CAD build for the part. Positions are in the model's coordinates, mm. Face numbers are marked on the shaded views. A direction names the side the tool comes from. Coordinates: 2 decimals unless noted, no trailing zeros. Loops run counter-clockwise (first coordinate to the right, second up) from the corner with the lowest first, then second, coordinate; pieces in that order, holes last. Notation, with made-up numbers: (67, 55) -> (103, 55) arc R18 cw to (103, 84) -> close; hole circle Ø2 at (7, 16). An arc over 180 degrees is marked (long way). Answer as a JSON object with one key per item and string values. Group by question number.
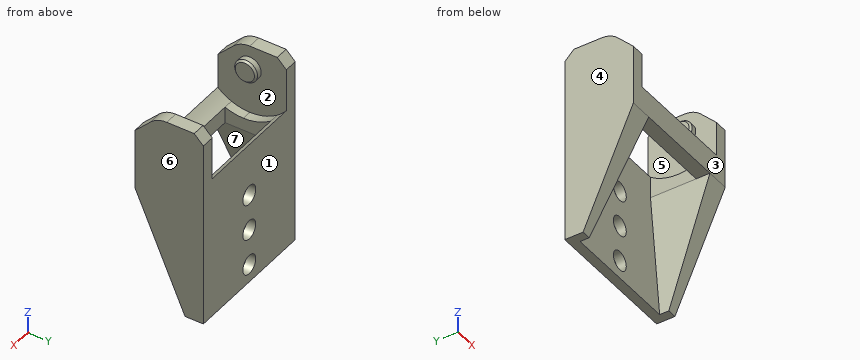
from build123d import *

# Parameters (mm, degrees)
SKETCH_1_W               = 30
SKETCH_1_H               = 15
EXTRUDE_1_DEPTH          = 18
CUT_EXTRUDE_1_REACH      = 28.843
SKETCH_2_W               = 20
SKETCH_2_H               = 10
CUT_EXTRUDE_2_REACH      = 29.668
SKETCH_3_W               = 20
SKETCH_3_H               = 12
CUT_EXTRUDE_5_DEPTH      = 22.1
CUT_EXTRUDE_5_DEPTH_BACK = 2.1
SKETCH_4_W               = 5
SKETCH_4_H               = 6
SKETCH_5_R               = 2.5
EXTRUDE_2_DEPTH          = 1.6
EXTRUDE_START            = 1.6
SKETCH_6_R               = 2.5
EXTRUDE_3_DEPTH          = 1.6
CHAMFER_1_SIZE           = 0.4
CUT_EXTRUDE_6_DEPTH      = 35.020684023
CUT_EXTRUDE_6_DEPTH_BACK = 35.020684023
CUT_EXTRUDE_7_DEPTH      = 35.020684023
CUT_EXTRUDE_7_DEPTH_BACK = 35.020684023
CHAMFER_2_SIZE           = 2
EXTRUDE_4_DEPTH          = 25
CHAMFER_3_SIZE           = 25
CHAMFER_3_SIZE2          = 11
SKETCH_10_R              = 2.1
CUT_EXTRUDE_8_DEPTH      = 15
CHAMFER_4_SIZE           = 3
CHAMFER_4_SIZE_2         = 25


with BuildPart() as part:
    # 草圖1 → 填料-伸長1 (new body)
    with BuildSketch(Plane.XY):
        with Locations((2.249045701, -2.44972067)):
            Rectangle(SKETCH_1_W, SKETCH_1_H)
    extrude(amount=EXTRUDE_1_DEPTH)

    # 草圖2 → 除料-伸長1 (cut, up to next)
    with BuildSketch(Plane.XY.offset(18), mode=Mode.PRIVATE) as cut_extrude_1_sk1:
        with Locations((2.249045701, -1.94972067)):
            Rectangle(SKETCH_2_W, SKETCH_2_H)
    cut_extrude_1_tool1 = extrude(cut_extrude_1_sk1.sketch, amount=-CUT_EXTRUDE_1_REACH, mode=Mode.PRIVATE) & part.part
    add(cut_extrude_1_tool1.solids().sort_by_distance((2.249046, -1.949721, 18))[0], mode=Mode.SUBTRACT)

    # 草圖3 → 除料-伸長2 (cut, up to next)
    with BuildSketch(Plane(origin=(0, -6.94972067, 0), x_dir=(1, 0, 0), z_dir=(0, 1, 0)), mode=Mode.PRIVATE) as cut_extrude_2_sk1:
        with Locations((2.249045701, -12)):
            Rectangle(SKETCH_3_W, SKETCH_3_H)
    cut_extrude_2_tool1 = extrude(cut_extrude_2_sk1.sketch, amount=-CUT_EXTRUDE_2_REACH, mode=Mode.PRIVATE) & part.part
    add(cut_extrude_2_tool1.solids().sort_by_distance((2.249046, -6.949721, 12))[0], mode=Mode.SUBTRACT)

    # 草圖4 → 除料-伸長5 (cut, two sides: drawn at the far end of the back side and taken through both)
    with BuildSketch(Plane(origin=(-7.750954299, 0, 0), x_dir=(0, 0, -1), z_dir=(1, 0, 0)).offset(-CUT_EXTRUDE_5_DEPTH_BACK)):
        with Locations((-15.5, 0.05027933)):
            Rectangle(SKETCH_4_W, SKETCH_4_H)
        with BuildLine():
            Line((-13, 3.05027933), (-13, -2.94972067))
            Line((-13, -2.94972067), (-18, -2.94972067))
            Line((-18, -2.94972067), (-18, -9.94972067))
            Line((-18, -9.94972067), (-6, -9.94972067))
            Line((-6, -9.94972067), (-6, -6.94972067))
            Line((-6, -6.94972067), (-3.562706956, -6.94972067))
            ThreePointArc((-3.562706956, -6.94972067), (-2.955231369, -4.990584005), (-2.75, -2.94972067))
            ThreePointArc((-2.75, -2.94972067), (-3.246950555, 0.203139384), (-4.689614931, 3.05027933))
            Line((-4.689614931, 3.05027933), (-13, 3.05027933))
        make_face()
        with BuildLine():
            ThreePointArc((-18, 5.998044414), (-15.583399687, 6.969379392), (-13, 7.30027933))
            Line((-13, 7.30027933), (-13, 7.89449882))
            Line((-13, 7.89449882), (-18, 7.89449882))
            Line((-18, 7.89449882), (-18, 5.998044414))
        make_face()
        with BuildLine():
            Line((-13, 7.30027933), (-13, 3.05027933))
            Line((-13, 3.05027933), (-4.689614931, 3.05027933))
            ThreePointArc((-4.689614931, 3.05027933), (-8.332961324, 6.176135454), (-13, 7.30027933))
        make_face()
        with BuildLine():
            Line((-18, 3.05027933), (-13, 3.05027933))
            Line((-13, 3.05027933), (-13, 7.30027933))
            ThreePointArc((-13, 7.30027933), (-15.583399687, 6.969379392), (-18, 5.998044414))
            Line((-18, 5.998044414), (-18, 3.05027933))
        make_face()
        with BuildLine():
            Line((-18, -9.94972067), (-18, -2.94972067))
            Line((-18, -2.94972067), (-18, 3.05027933))
            Line((-18, 3.05027933), (-18, 5.998044414))
            ThreePointArc((-18, 5.998044414), (-19.843504041, -10.580510436), (-3.562706956, -6.94972067))
            Line((-3.562706956, -6.94972067), (-6, -6.94972067))
            Line((-6, -6.94972067), (-6, -9.94972067))
            Line((-6, -9.94972067), (-18, -9.94972067))
        make_face()
    extrude(amount=CUT_EXTRUDE_5_DEPTH + CUT_EXTRUDE_5_DEPTH_BACK, mode=Mode.SUBTRACT)

    # 草圖5 → 填料-伸長2 (add)
    with BuildSketch(Plane.ZY.offset(-14.349045701)):
        with Locations(Location((13, -2.94972067, 0), (0, 0, 90))):
            Circle(SKETCH_5_R)
    extrude(amount=EXTRUDE_2_DEPTH)

    # 草圖6 → 填料-伸長3 (add)
    with BuildSketch(Plane(origin=(-9.850954299, 0, 0), x_dir=(0, 0, -1), z_dir=(1, 0, 0)).offset(EXTRUDE_START)):
        with Locations(Location((-13, -2.94972067, 0), (0, 0, 90))):
            Circle(SKETCH_6_R)
    extrude(amount=-EXTRUDE_3_DEPTH)

    # 導角1
    chamfer_1_edges = [part.edges().sort_by_distance(p)[0] for p in [
        (12.749045701, -5.44972067, 13),
        (-8.250954299, -5.44972067, 13),
    ]]
    chamfer(chamfer_1_edges, length=CHAMFER_1_SIZE)

    # 草圖7 → 除料-伸長6 (cut, two sides: drawn at the far end of the back side and taken through both)
    with BuildSketch(Plane(origin=(-9.850954299, 0, 0), x_dir=(0, 0, -1), z_dir=(1, 0, 0)).offset(-CUT_EXTRUDE_6_DEPTH_BACK)):
        Polygon((-18, -9.94972067), (-13.071067812, -9.94972067), (-18, -5.020788482), align=None)
    extrude(amount=CUT_EXTRUDE_6_DEPTH + CUT_EXTRUDE_6_DEPTH_BACK, mode=Mode.SUBTRACT)

    # 草圖8 → 除料-伸長7 (cut, two sides: drawn at the far end of the back side and taken through both)
    with BuildSketch(Plane(origin=(-9.850954299, 0, 0), x_dir=(0, 0, -1), z_dir=(1, 0, 0)).offset(-CUT_EXTRUDE_7_DEPTH_BACK)):
        with BuildLine():
            Line((-18, -2.94972067), (-18, -5.020788482))
            Line((-18, -5.020788482), (-16.535533871, -6.485254612))
            ThreePointArc((-16.535533871, -6.485254612), (-17.619397653, -4.863137855), (-18, -2.94972067))
        make_face()
    extrude(amount=CUT_EXTRUDE_7_DEPTH + CUT_EXTRUDE_7_DEPTH_BACK, mode=Mode.SUBTRACT)

    # 導角2
    chamfer_2_edges = [part.edges().sort_by_distance(p)[0] for p in [
        (15.799045701, 5.05027933, 18),
        (-11.300954299, 5.05027933, 18),
    ]]
    chamfer(chamfer_2_edges, length=CHAMFER_2_SIZE)

    # 草圖9 → 填料-伸長4 (add)
    with BuildSketch(Plane(origin=(0, 0, 0), x_dir=(-1, 0, 0), z_dir=(0, 0, -1))):
        Polygon((-12.249045701, 3.05027933), (-12.249045701, -9.94972067), (-17.249045701, -9.94972067), (-17.249045701, 5.05027933), (12.750954299, 5.05027933), (12.750954299, -9.94972067), (7.750954299, -9.94972067), (7.750954299, 3.05027933), align=None)
    extrude(amount=EXTRUDE_4_DEPTH)

    # 導角3
    chamfer_3_edges = [part.edges().sort_by_distance(p)[0] for p in [
        (-10.250954299, -9.94972067, -25),
        (14.749045701, -9.94972067, -25),
    ]]
    chamfer_3_side = [part.faces().sort_by_distance(p)[0] for p in [
        (2.249045701, -9.94972067, 0.484706737),
    ]]
    chamfer(chamfer_3_edges, length=CHAMFER_3_SIZE, length2=CHAMFER_3_SIZE2, reference=chamfer_3_side[0])

    # 草圖10 → 除料-伸長8 (cut)
    with BuildSketch(Plane.XZ.offset(-3.05027933)):
        with Locations(Location((2.249045701, -21, 0), (0, 0, 270))):
            Circle(SKETCH_10_R)
        with Locations(Location((2.249045701, -13, 0), (0, 0, 270))):
            Circle(SKETCH_10_R)
        with Locations(Location((2.249045701, -5, 0), (0, 0, 270))):
            Circle(SKETCH_10_R)
    extrude(amount=-CUT_EXTRUDE_8_DEPTH, mode=Mode.SUBTRACT)

    # 導角4
    # the kernel refuses this chamfer: 25, 3 mm, written as the material it takes off along each edge
    with BuildSketch(Plane(origin=(-7.750954299, -63.93259543, -25), x_dir=(-0.952888564534268, 0, -0.3033205953769419), z_dir=(0, 1, 0)), Plane(origin=(12.249045701, 3.05027933, -25), x_dir=(0.952888564534268, 0, -0.3033205953769419), z_dir=(0, -1, 0))) as chamfer_4_piece_1:
        Polygon((CHAMFER_4_SIZE * 0.952888564534, CHAMFER_4_SIZE * 0.303320595377), (-CHAMFER_4_SIZE_2 * 0.303320595377, CHAMFER_4_SIZE_2 * 0.952888564534), (0, 0), align=None)
    extrude(amount=66.98287476, mode=Mode.SUBTRACT)


solid = part.part
Item 1: Band-saw the part on D-D, the plane z = -21. List the corners of the cut face in (x, y), and give its area (3 significant figures).
Item 2: 3-axis set-ups, long thin cutter, end or side, ignore diameter. For the marked faces 5, 6 and 7: which of +Z, -Z, +X, -X, +Y, -Y reach the whole face in a straight line?
Item 3: Band-saw the part on A-A, the plane x = -2. List the corners of the cut face in (y, z), and give its area (3 significant figures).
Item 4: Band-saw the part on B-B, the plane z = -5. List the corners of the cut face in (x, y), and give its area (3 significant figures).
Item 5: Drill centre lines: L1, parallel to X at y = 4.5, z = -5; L2, parallel to X at y = -6.25, z = 6; L3, parallel to Y at x = 6.5, z = -13. Where is each one in solid material? Low to high.
Item 6: Flat gauge pins, fed straight in: P1, Ø0.9, axis at x = 4, y = -9, coming from the -Z side; P2, Ø8, axis at x = -1, z = -6, coming from the -Y side; P3, Ø3, axis at x = -5.5, y = -7.5, coming from the +Z side. Where does each tip first touch, or does it go through?
Item 7: Pull direction Y, two halves, no side cores. Call the marked faces 1, 2, 3 and 4: +Y half, -Y half, draft (parallel to the pull), parting line (faces both ways), or undercut.
Item 8: Band-saw the part on C-C, the plane z = -16. List the corners of the cut face in (x, y).
Reply:
{
 "1": {"outline": "(-12.75, -0.71) -> (-10.27, -0.71) -> (-10.27, 3.05) -> (0.15, 3.05) -> (0.15, 5.05) -> (-12.75, 5.05) -> close; (4.35, 3.05) -> (14.77, 3.05) -> (14.77, -0.71) -> (17.25, -0.71) -> (17.25, 5.05) -> (4.35, 5.05) -> close", "area": "70.2 mm²"},
 "2": {"face 5": "none", "face 6": "+Z, -Z, +X, +Y, -Y", "face 7": "-Z, -Y"},
 "3": {"outline": "(-9.95, 0) -> (-6.95, 0) -> (-6.95, 3.56) arc R10.25 cw to (-9.95, 5.51) -> close; (3.05, -25) -> (5.05, -25) -> (5.05, 6.59) arc R10.25 cw to (3.05, 4.69) -> close", "area": "74.3 mm²"},
 "4": {"outline": "(-12.75, -7.75) -> (-8.35, -7.75) -> (-8.35, 3.05) -> (0.15, 3.05) -> (0.15, 5.05) -> (-12.75, 5.05) -> close; (4.35, 3.05) -> (12.85, 3.05) -> (12.85, -7.75) -> (17.25, -7.75) -> (17.25, 5.05) -> (4.35, 5.05) -> close", "area": "147 mm²"},
 "5": {"L1": "-12.75 to 0.15, 4.35 to 17.25", "L2": "-12.75 to -9.85, 14.35 to 17.25", "L3": "3.05 to 5.05"},
 "6": {"P1": "z = 0", "P2": "y = 3.05", "P3": "z = 4.73"},
 "7": {"face 1": "+Y half", "face 2": "undercut", "face 3": "-Y half", "face 4": "draft"},
 "8": {"outline": "(-12.75, -2.91) -> (-9.67, -2.91) -> (-9.67, 3.05) -> (14.17, 3.05) -> (14.17, -2.91) -> (17.25, -2.91) -> (17.25, 5.05) -> (-12.75, 5.05) -> close"}
}
